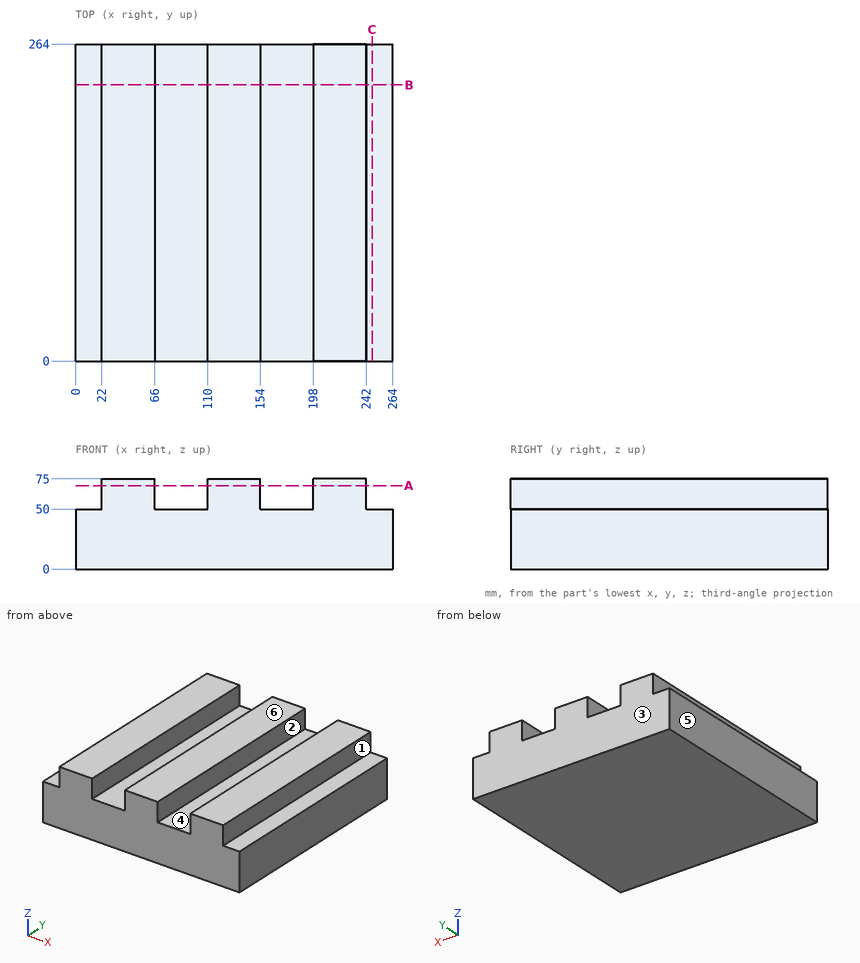
Drawing for the job (mm, zero at the part's lowest x, y, z). A direction names the side the tool comes from. Round coordinates to 2 decimals unless told otherwise and drop trailing zeros. Loops run counter-clockwise (first coordinate to the right, second up) from the corner with the lowest first, then second, coordinate; pieces in that order, holes last. Notation, with made-up numbers: (59.5, 76) -> (88.5, 76) arc R16 ccw to (88.5, 80) -> close; hole circle Ø2 at (-31.5, 31). An arc over 180 degrees is marked (long way). Answer as CSV lines item,"result". Start each with the question number.
1) Mould opens along X. For the marked faces 4, 5 and 6 say: +X half, -X half, draft (parallel to the pull), parting line (faces both ways), or undercut.
2) Slice it at C-C (x = 247). List the corners of the cut face in (y, z), plus the area to 3 significant figures.
3) Slice it at B-B (y = 230). List the corners of the cut face in (x, z), plus the area to 3 significant figures.
4) Tool access for the marked faces 1, 2 and 3: list every direction of +Z, -Z, +X, -X, +Y, -Y with a clear straight run to the whole face (end or side of a thin tool).
5) Slice it at A-A (z = 69.5). List the corners of the cut face in (x, y), plus the area to 3 significant figures.
6) Pin check, flat tips, straight feed: P1, Ø12.5, axis at y = 73.5, z = 68.5, coming from the +X side; P2, Ø17.5, axis at x = 10, y = 125.5, coming from the +Z side. Stop position of each tip, or through.
7) Probe line 1 along X through (y, z) = (45.5, 58); line 2 along Z through (x, y) = (93.5, 253.5). List the from-to ranges inside material, lowest first.
Filled in:
1,face 4,"undercut"
1,face 5,"-X half"
1,face 6,"draft"
2,outline,"(0, 0) -> (264, 0) -> (264, 50) -> (0, 50) -> close"
2,area,"13,200 mm2"
3,outline,"(0, 0) -> (264, 0) -> (264, 50) -> (242, 50) -> (242, 75) -> (198, 75) -> (198, 50) -> (154, 50) -> (154, 75) -> (110, 75) -> (110, 50) -> (66, 50) -> (66, 75) -> (22, 75) -> (22, 50) -> (0, 50) -> close"
3,area,"16,500 mm2"
4,face 1,"+Z, +X, +Y, -Y"
4,face 2,"+Z, +Y, -Y"
4,face 3,"+Z, -Z, +X, -X, +Y"
5,outline,"(22, 0) -> (66, 0) -> (66, 264) -> (22, 264) -> close; (110, 0) -> (154, 0) -> (154, 264) -> (110, 264) -> close; (198, 0) -> (242, 0) -> (242, 264) -> (198, 264) -> close"
5,area,"34,800 mm2"
6,P1,"stops at x = 242"
6,P2,"stops at z = 50"
7,line 1,"x = 22 to 66, 110 to 154, 198 to 242"
7,line 2,"z = 0 to 50"
